Read the model definition and answer for the solid it produces. Units are mm, in the model's axes. A direction names the side the tool comes from. Round coordinates to 2 decimals unless told otherwise and drop trailing zeros. Order: outer loops, then holes, each group sorted by start corner. A loop starts at its lowest first (then second) coordinate and runs counter-clockwise, first axis right, second up. Notation, with made-up numbers: M -5.5,41.25 L 27.5,41.25 A37 ccw 27.5,79.25 Z; hole C 49.5,-37.75 d2. An arc over 180 degrees is marked long. Answer as CSV lines item,"result".
```python
from build123d import *

# Parameters (mm, degrees)
SKETCH1_W           = 160
SKETCH1_H           = 53
BOSS_EXTRUDE1_DEPTH = 76
SKETCH2_W           = 156
SKETCH2_H           = 49
CUT_EXTRUDE1_DEPTH  = 74
CUT_EXTRUDE2_REACH  = 4
SKETCH3_R           = 2
SKETCH4_W           = 30
SKETCH4_H           = 2
SKETCH4_W_2         = 20
SKETCH4_H_2         = 20
CUT_EXTRUDE3_DEPTH  = 74


with BuildPart() as part:
    # Sketch1 → Boss-Extrude1 (new body)
    with BuildSketch(Plane.XY):
        Rectangle(SKETCH1_W, SKETCH1_H)
    extrude(amount=BOSS_EXTRUDE1_DEPTH)

    # Sketch2 → Cut-Extrude1 (cut)
    with BuildSketch(Plane.XY.offset(76)):
        Rectangle(SKETCH2_W, SKETCH2_H)
    extrude(amount=-CUT_EXTRUDE1_DEPTH, mode=Mode.SUBTRACT)

    # Sketch3 → Cut-Extrude2 (cut, up to next)
    with BuildSketch(Plane.XY.offset(2), mode=Mode.PRIVATE) as cut_extrude2_sk1:
        with Locations((50, 0)):
            Circle(SKETCH3_R)
    cut_extrude2_tool1 = extrude(cut_extrude2_sk1.sketch, amount=-CUT_EXTRUDE2_REACH, mode=Mode.PRIVATE) & part.part
    add(cut_extrude2_tool1.solids().sort_by_distance((50, 0, 2))[0], mode=Mode.SUBTRACT)
    # Sketch3 → Cut-Extrude2 (cut, up to next)
    with BuildSketch(Plane.XY.offset(2), mode=Mode.PRIVATE) as cut_extrude2_sk2:
        with Locations((-50, 0)):
            Circle(SKETCH3_R)
    cut_extrude2_tool2 = extrude(cut_extrude2_sk2.sketch, amount=-CUT_EXTRUDE2_REACH, mode=Mode.PRIVATE) & part.part
    add(cut_extrude2_tool2.solids().sort_by_distance((-50, 0, 2))[0], mode=Mode.SUBTRACT)

    # Sketch4 → Cut-Extrude3 (cut)
    with BuildSketch(Plane.XY.offset(76)):
        with Locations((0, 25.5)):
            Rectangle(SKETCH4_W, SKETCH4_H)
        with Locations((0, -25.5)):
            Rectangle(SKETCH4_W, SKETCH4_H)
        with Locations((80, -25)):
            Rectangle(SKETCH4_W_2, SKETCH4_H_2)
    extrude(amount=-CUT_EXTRUDE3_DEPTH, mode=Mode.SUBTRACT)


solid = part.part
```
Item 1: Flat-ended cylindrical pins translate along their axes: pin 1 (2.5 mm diameter, centred on x = 50, y = 0, fed in from -Z); pin 2 (0.6 mm diameter, centred on x = 79.5, z = 34.5, fed in from -Y); pin 3 (2 mm diameter, centred on y = -25.5, z = 45.5, fed in from +X); pin 4 (5 mm diameter, centred on x = -50, y = 0, fed in from +Z). Find the tip coordinate at first contact, or state that the pin passes through.
Ans:
pin 1,"through"
pin 2,"y = -15"
pin 3,"x = 70"
pin 4,"z = 2"
Item 2: A cutting plane is placed at A-A, the plane x = 50. Determine the outline of the cut face in (y, z), and give its area (3 significant figures).
Ans:
outline,"M -26.5,0 L -2,0 L -2,2 L -24.5,2 L -24.5,76 L -26.5,76 Z; M 2,0 L 26.5,0 L 26.5,76 L 24.5,76 L 24.5,2 L 2,2 Z"
area,"394 mm2"
Item 3: A cutting plane is placed at D-D, the plane y = -23. Determine the outline of the cut face in (x, z).
Ans:
outline,"M -80,0 L 80,0 L 80,2 L -78,2 L -78,76 L -80,76 Z"
Item 4: Find the intervals of material crossed by probe 1 along X at (y, z) = (-9, 46.5); probe 2 along Y at (x, z) = (-55, 17); probe 3 along Y at (x, z) = (50, 0.85), in increasing order. Write a range as [from, to].
Ans:
probe 1,"[-80, -78], [78, 80]"
probe 2,"[-26.5, -24.5], [24.5, 26.5]"
probe 3,"[-26.5, -2], [2, 26.5]"
Item 5: A cutting plane is placed at C-C, the plane z = 27. Determine the outline of the cut face in (x, y).
Ans:
outline,"M -80,-26.5 L -15,-26.5 L -15,-24.5 L -78,-24.5 L -78,24.5 L -15,24.5 L -15,26.5 L -80,26.5 Z; M 15,-26.5 L 70,-26.5 L 70,-24.5 L 15,-24.5 Z; M 15,24.5 L 78,24.5 L 78,-15 L 80,-15 L 80,26.5 L 15,26.5 Z"
Item 6: A tool of negligible diameter and unlimited length cuts with its end or side. For faces 4 (the face through (42, -24.5, 40)), 5 (the face through (-78, 0, 40)), 6 (the face through (78, 4, 40)), from which of +Z, -Z, +X, -X, +Y, -Y can it reach the whole face along a straight path? Write none if from no direction.
Ans:
face 4,"+Z, +X"
face 5,"+Z"
face 6,"+Z, -Y"
Item 7: A cutting plane is placed at B-B, the plane y = 0. Determine the outline of the cut face in (x, z), and give its area (3 significant figures).
Ans:
outline,"M -80,0 L -52,0 L -52,2 L -78,2 L -78,76 L -80,76 Z; M -48,0 L 48,0 L 48,2 L -48,2 Z; M 52,0 L 80,0 L 80,76 L 78,76 L 78,2 L 52,2 Z"
area,"600 mm2"
Item 8: Determine the mould class of faces 1 (the face through (-47, -24.5, 40)), 2 (the face through (62, 26, 76)), 3 (the face through (-19, -26.5, 37)) for opening direction Y: +Y half, -Y half, draft (parallel to the pull), parting line (faces both ways), or undercut.
Ans:
face 1,"undercut"
face 2,"draft"
face 3,"-Y half"
